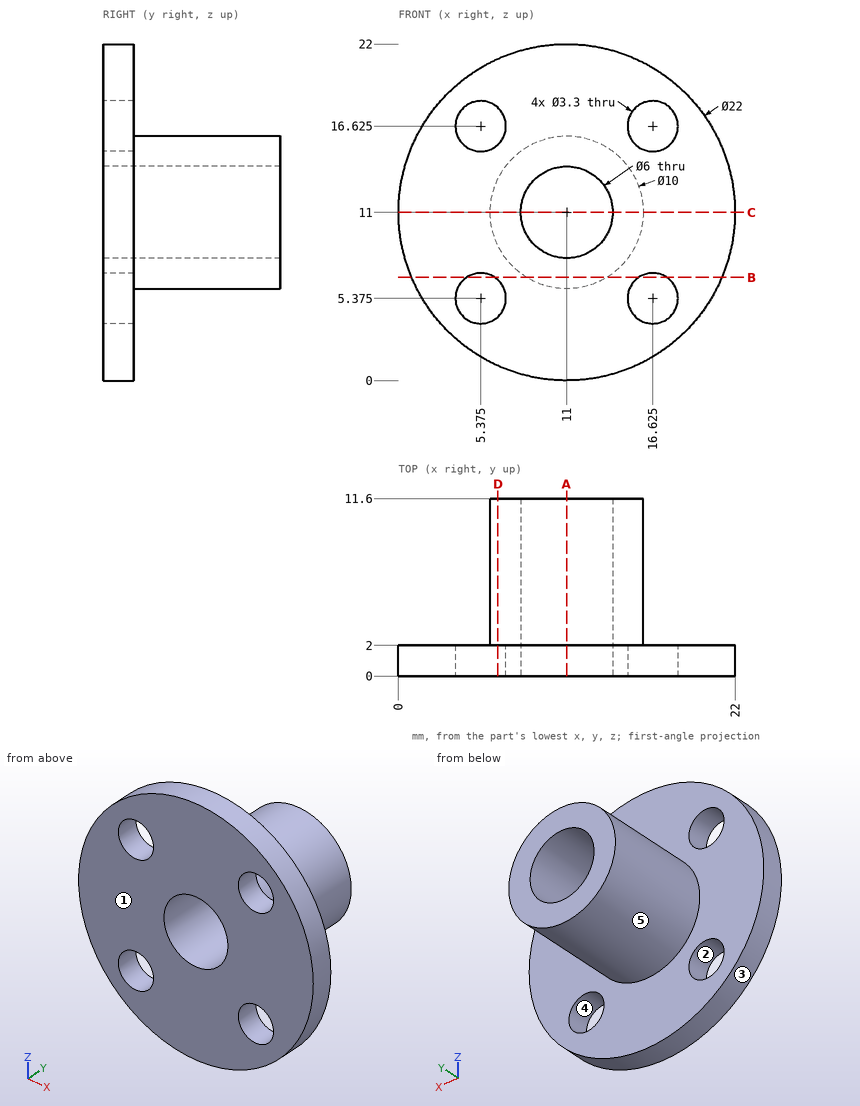
Verification items for this drawing (mm, ordinates from the low corner). A direction names the side the tool comes from. Give positions to 0.01 mm unless a question says otherwise; leave off trailing zeros. Write each loop counter-clockwise with the first axis right and the second up, starting at its lowest first coordinate (ties: lowest second). Pieces come first, ordered by that corner, then holes.
1) Cross-section at D-D (x = 6.5). Record the boundary of the cut face in (y, z), plus the area to 3 significant figures.
Values follow:
outline: (0, 0.96) - (2, 0.96) - (2, 4.17) - (0, 4.17) - close; (0, 6.58) - (2, 6.58) - (2, 8.82) - (11.6, 8.82) - (11.6, 13.18) - (2, 13.18) - (2, 15.42) - (0, 15.42) - close; (0, 17.83) - (2, 17.83) - (2, 21.04) - (0, 21.04) - close
area: 72.3 mm2
2) Set-up check for the marked faces 4 and 5: record each of +Z, -Z, +X, -X, +Y, -Y from which the full face is reachable in a straight line by a thin tool's end or side.
Values follow:
face 4: +Y, -Y
face 5: +Y
3) Cross-section at C-C (z = 11). Record the boundary of the cut face in (x, y).
Values follow:
outline: (0, 0) - (8, 0) - (8, 11.6) - (6, 11.6) - (6, 2) - (0, 2) - close; (14, 0) - (22, 0) - (22, 2) - (16, 2) - (16, 11.6) - (14, 11.6) - close
4) Go/stop test with flat-tipped pins: pin 1 Ø3 at (x, z) = (16.625, 5.375) entering from -Y; pin 2 Ø4 at (y, z) = (1.5, 3) entering from -X; pin 3 Ø3 at (x, z) = (18.5, 8) entering from +Y. Record where each tip stops, or that it passes through.
Values follow:
pin 1: passes through
pin 2: stops at x = 1.78
pin 3: stops at y = 2
5) Release check for a two-part mould opening along Z. For the marked faces 1, 2 and 3 record: released by +Z, released by -Z, zero draft, split by the parting line, or undercut.
Values follow:
face 1: zero draft
face 2: undercut
face 3: split by the parting line
6) Cross-section at B-B (z = 6.75). Record the boundary of the cut face in (x, y), plus the area to 3 significant figures.
Values follow:
outline: (0.85, 0) - (4.46, 0) - (4.46, 2) - (0.85, 2) - close; (6.29, 0) - (15.71, 0) - (15.71, 2) - (13.63, 2) - (13.63, 11.6) - (8.37, 11.6) - (8.37, 2) - (6.29, 2) - close; (17.54, 0) - (21.15, 0) - (21.15, 2) - (17.54, 2) - close
area: 83.9 mm2
7) Cross-section at A-A (x = 11). Record the boundary of the cut face in (y, z).
Values follow:
outline: (0, 0) - (2, 0) - (2, 6) - (11.6, 6) - (11.6, 8) - (0, 8) - close; (0, 14) - (11.6, 14) - (11.6, 16) - (2, 16) - (2, 22) - (0, 22) - close
8) Thickness scan on line 1 (Y direction, x = 19.5, z = 7.5); line 2 (X direction, y = 7.25, z = 9.75); line 3 (X direction, y = 1.5, z = 13.5). Record the ranges inside material, lowest first.
Values follow:
line 1: y = 0 to 2
line 2: x = 6.16 to 8.27, 13.73 to 15.84
line 3: x = 0.29 to 9.34, 12.66 to 21.71
